Here's how the part is built. I have some questions about the finished solid (model axes, mm). Face numbers are marked on the shaded views. Give positions to 0.01 mm unless a question says otherwise; leave off trailing zeros. Loops run counter-clockwise (first coordinate to the right, second up) from the corner with the lowest first, then second, coordinate; pieces in that order, holes last.
Q1. I need wall thicknesses on line 1 (Y direction, x = 14.5, z = 1.65); line 2 (Y direction, x = -14.2, z = 1.8); line 3 (Y direction, x = 0, z = 2.55). Which ranges of each line are inside material? Lowest first, please.
Q2. If we section it at C-C (x = -14.2): Please give me the cut outline in (y, z).
Q3. If we section it at B-B (y = 10): Please give me the cut outline in (x, z), plus the area to 3 significant figures.
Q4. If we section it at D-D (y = 0): Please give me the cut outline in (x, z) (3 decimals), plus the area to 3 significant figures.
Q5. If we section it at A-A (x = 14.5): Please give me the cut outline in (y, z).
Q6. We'd pull the mould along Z, two halves only. Please class the marked faces 1, 2 and 3: +Z half, -Z half, draft (parallel to the pull), parting line (faces both ways), or undercut.
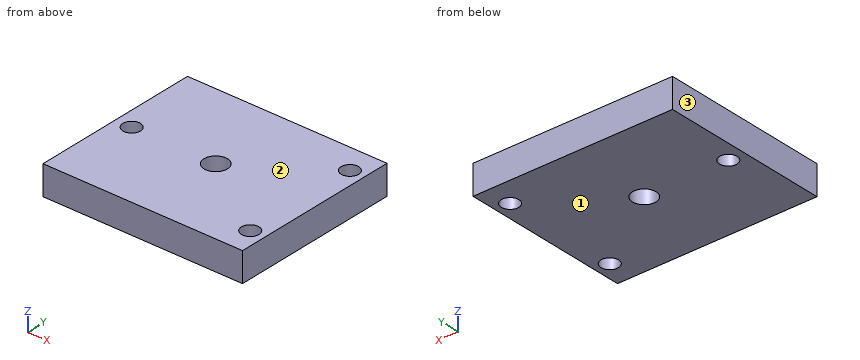
Autodesk Inventor part; units mm, degrees
ref_plane "YZ Plane" through (0, 0, 0) normal (1, 0, 0) x (0, 1, 0)
ref_plane "XZ Plane" through (0, 0, 0) normal (0, 1, 0) x (-1, 0, 0)
ref_plane "XY Plane" through (0, 0, 0) normal (0, 0, 1) x (1, 0, 0)
sketch "Sketch1" plane through (0, 0, 0) normal (0, 0, 1) x (1, 0, 0)
  point P0 (0, 0)
sketch "Sketch2" plane through (0, 0, 0) normal (0, 0, 1) x (1, 0, 0)
  line L0 (-17, -14.5) -> (17, -14.5)
  line L1 (17, -14.5) -> (17, 14.5)
  line L2 (17, 14.5) -> (-17, 14.5)
  line L3 (-17, 14.5) -> (-17, -14.5)
  circle A0 centre (14.5, 10) radius 1.5
  circle A1 centre (14.5, -10) radius 1.5
  circle A2 centre (-14.2, 0) radius 1.5
  point P0 (0, 0)
  dimension "d0" = 34
  dimension "d1" = 29
  dimension "d2" = 3
  dimension "d3" = 3
  dimension "d4" = 3
  dimension "d5" = 20
  dimension "d6" = 2.5
  dimension "d7" = 14.5
  dimension "d8" = 28.7
extrude "Extrusion1" add sketch "Sketch2" along normal blind 5
thread "Thread1"
thread "Thread2"
thread "Thread3"
sketch "Sketch3" plane through (0, 0, 5) normal (0, 0, 1) x (1, 0, 0)
  line L0 (-7.3481, 13.6395) -> (7.272, 13.6395) construction
  line L1 (7.272, 13.6395) -> (7.272, 4.876) construction
  line L2 (7.272, 4.876) -> (-7.3481, 4.876) construction
  line L3 (-7.3481, 4.876) -> (-7.3481, 13.6395) construction
  point P0 (0, 0)
  dimension "d0" = 34
  dimension "d1" = 29
  dimension "d2" = 3
  dimension "d3" = 3
  dimension "d4" = 3
  dimension "d5" = 20
  dimension "d6" = 2.5
  dimension "d7" = 14.5
  dimension "d8" = 28.7
sketch "Sketch4" plane through (0, 0, 5) normal (0, 0, 1) x (1, 0, 0)
  circle A0 centre (0.125, 0) radius 2
  circle A1 centre (14.5, 10) radius 1.5
  circle A2 centre (-14.2, 0) radius 1.5
  dimension "d18" = 4
  dimension "d21" = 14.375
extrude "Extrusion2" cut sketch "Sketch4" against normal blind 5 contours A0
thread "Thread4"
properties material "ABS Plastic"
Check sheet entries:
1. line 1: y = -14.5 to -11.5, -8.5 to 8.5, 11.5 to 14.5
1. line 2: y = -14.5 to -1.5, 1.5 to 14.5
1. line 3: y = -14.5 to -2, 2 to 14.5
2. outline: (-14.5, 0) - (-1.5, 0) - (-1.5, 5) - (-14.5, 5) - close; (1.5, 0) - (14.5, 0) - (14.5, 5) - (1.5, 5) - close
3. outline: (-17, 0) - (13, 0) - (13, 5) - (-17, 5) - close; (16, 0) - (17, 0) - (17, 5) - (16, 5) - close
3. area: 155 mm2
4. outline: (-17, 0) - (-15.7, 0) - (-15.7, 5) - (-17, 5) - close; (-12.7, 0) - (-1.875, 0) - (-1.875, 5) - (-12.7, 5) - close; (2.125, 0) - (17, 0) - (17, 5) - (2.125, 5) - close
4. area: 135 mm2
5. outline: (-14.5, 0) - (-11.5, 0) - (-11.5, 5) - (-14.5, 5) - close; (-8.5, 0) - (8.5, 0) - (8.5, 5) - (-8.5, 5) - close; (11.5, 0) - (14.5, 0) - (14.5, 5) - (11.5, 5) - close
6. face 1: -Z half
6. face 2: +Z half
6. face 3: draft
